```python
from build123d import *

# Parameters (mm, degrees)
SKETCH1_R           = 7.5
BOSS_EXTRUDE5_DEPTH = 20
SKETCH2_R           = 7.5
BOSS_EXTRUDE6_DEPTH = 35
SKETCH3_W           = 17.737554882
SKETCH3_H           = 20
BOSS_EXTRUDE7_DEPTH = 30


with BuildPart() as part:
    # Sketch1 → Boss-Extrude5 (new body)
    # profile 1 of 6: a face of its own
    with BuildSketch(Plane.XY):
        with BuildLine():
            ThreePointArc((133.138593384, 0), (130, 10), (133.138593384, 20))
            Line((133.138593384, 20), (0, 20))
            Line((0, 20), (0, 10))
            Line((0, 10), (0, 0))
            Line((0, 0), (133.138593384, 0))
        make_face()
        with BuildLine():
            ThreePointArc((15, 10), (7.5, 2.5), (0, 10))
            ThreePointArc((0, 10), (7.5, 17.5), (15, 10))
        make_face(mode=Mode.SUBTRACT)
    # profile 2 of 6: a face of its own
    with BuildSketch(Plane.XY):
        with BuildLine():
            ThreePointArc((147.5, 2.5), (140, 10), (147.5, 17.5))
            Line((147.5, 17.5), (147.5, 20))
            Line((147.5, 20), (133.138593384, 20))
            ThreePointArc((133.138593384, 20), (130, 10), (133.138593384, 0))
            Line((133.138593384, 0), (147.5, 0))
            Line((147.5, 0), (147.5, 2.5))
        make_face()
    # profile 3 of 6: a face of its own
    with BuildSketch(Plane.XY):
        with BuildLine():
            Line((147.5, 20), (147.5, 17.5))
            ThreePointArc((147.5, 17.5), (152.803300859, 15.303300859), (155, 10))
            ThreePointArc((155, 10), (152.803300859, 4.696699141), (147.5, 2.5))
            Line((147.5, 2.5), (147.5, 0))
            Line((147.5, 0), (133.138593384, 0))
            ThreePointArc((133.138593384, 0), (152.740485866, -6.696925103), (165, 10))
            ThreePointArc((165, 10), (152.740485866, 26.696925103), (133.138593384, 20))
            Line((133.138593384, 20), (147.5, 20))
        make_face()
    # profile 4 of 6: a face of its own
    with BuildSketch(Plane.XY):
        with Locations((7.5, 10)):
            Circle(SKETCH1_R)
    # profile 5 of 6: a face of its own
    with BuildSketch(Plane.XY):
        with BuildLine():
            ThreePointArc((147.5, 2.5), (140, 10), (147.5, 17.5))
            Line((147.5, 17.5), (147.5, 20))
            Line((147.5, 20), (133.138593384, 20))
            ThreePointArc((133.138593384, 20), (130, 10), (133.138593384, 0))
            Line((133.138593384, 0), (147.5, 0))
            Line((147.5, 0), (147.5, 2.5))
        make_face()
    # profile 6 of 6: a face of its own
    with BuildSketch(Plane.XY):
        with BuildLine():
            Line((147.5, 20), (147.5, 17.5))
            ThreePointArc((147.5, 17.5), (152.803300859, 15.303300859), (155, 10))
            ThreePointArc((155, 10), (152.803300859, 4.696699141), (147.5, 2.5))
            Line((147.5, 2.5), (147.5, 0))
            Line((147.5, 0), (133.138593384, 0))
            ThreePointArc((133.138593384, 0), (152.740485866, -6.696925103), (165, 10))
            ThreePointArc((165, 10), (152.740485866, 26.696925103), (133.138593384, 20))
            Line((133.138593384, 20), (147.5, 20))
        make_face()
    extrude(amount=BOSS_EXTRUDE5_DEPTH)

    # Sketch2 → Boss-Extrude6 (add)
    with BuildSketch(Plane(origin=(0, 0, 0), x_dir=(-1, 0, 0), z_dir=(0, 0, -1))):
        with Locations((-7.5, 10)):
            Circle(SKETCH2_R)
    extrude(amount=BOSS_EXTRUDE6_DEPTH)

    # Sketch3 → Boss-Extrude7 (add)
    with BuildSketch(Plane(origin=(0, 25, 0), x_dir=(1, 0, 0), z_dir=(0, 1, 0))):
        with Locations((147.498702773, -10)):
            Rectangle(SKETCH3_W, SKETCH3_H)
    extrude(amount=BOSS_EXTRUDE7_DEPTH)


solid = part.part
```
Input: part model. Units: mm. Frame: model coordinates. A direction names the side the tool comes from. Give positions to 0.01 mm unless a question says otherwise; leave off trailing zeros. Order: outer loops, then holes, each group sorted by start corner. A loop starts at its lowest first (then second) coordinate and runs counter-clockwise, first axis right, second up. Notation, with made-up numbers: (44, 4.5) -> (60, 4.5) arc R14 ccw to (60, 30.5) -> close; hole circle Ø7 at (43.5, 85). An arc over 180 degrees is marked (long way). Write each question's results on one line, items separated by ' | '. Start each with the question number.
Item 1: Contact query for flat-ended pins moving along their axis: P1, Ø10, axis at y = 26, z = -17, coming from the -X side; P2, Ø3, axis at y = 16, z = -27.5, coming from the -X side; P3, Ø2, axis at y = 13, z = -3.5, coming from the +X side; P4, Ø10, axis at x = 51, z = 10.5, coming from the +Y side. Output: stop coordinate, or through.
Item 2: Cut plane D-D on x = 7.5. Return the cut outline in (y, z).
Item 3: Cut plane A-A on z = 5.5. Return the cut outline in (x, y), then the cut area to 3 significant figures.
Item 4: Set-up query: faces 1 (the cylindrical face through (9.13, 2.68, -17.26)), 2 (the flat face through (66, 0, 10)), 3 (the flat face through (156.367, 40, 10)), 4 (the flat face through (68, 20, 10)). Return all of +Z, -Z, +X, -X, +Y, -Y with unobstructed straight access to the full face (end or side cutting, diameter ignored); none if empty.
Item 5: Line query: line 1 (Y direction, x = 147, z = 16.5); line 2 (Z direction, x = 123, y = 15.5). Output: solid intervals per line, ascending.
Item 6: Cut plane B-B on x = 141.5. Return the cut outline in (y, z).
Item 7: Cut plane C-C on y = 8.5. Return the cut outline in (x, z).
Established:
1) P1: through | P2: x = 1.5 | P3: x = 14.73 | P4: y = 20
2) outline: (0, 0) -> (2.5, 0) -> (2.5, -35) -> (17.5, -35) -> (17.5, 0) -> (20, 0) -> (20, 20) -> (0, 20) -> close
3) outline: (0, 0) -> (133.14, 0) arc R17.5 ccw (long way) to (156.37, 25.09) -> (156.37, 55) -> (138.63, 55) -> (138.63, 25.09) arc R17.5 ccw to (133.14, 20) -> (0, 20) -> close; hole circle Ø15 at (147.5, 10) | area: 3,910 mm^2
4) face 1: -Z | face 2: +Z, -Z, -X, -Y | face 3: +Z, -Z, +X, +Y | face 4: +Z, -Z, -X, +Y
5) line 1: -7.49 to 2.52, 17.48 to 55 | line 2: 0 to 20
6) outline: (-6.44, 0) -> (5.5, 0) -> (5.5, 20) -> (-6.44, 20) -> close; (14.5, 0) -> (55, 0) -> (55, 20) -> (14.5, 20) -> close
7) outline: (0, 0) -> (0.15, 0) -> (0.15, -35) -> (14.85, -35) -> (14.85, 0) -> (140.15, 0) -> (140.15, 20) -> (0, 20) -> close; (154.85, 0) -> (164.94, 0) -> (164.94, 20) -> (154.85, 20) -> close
